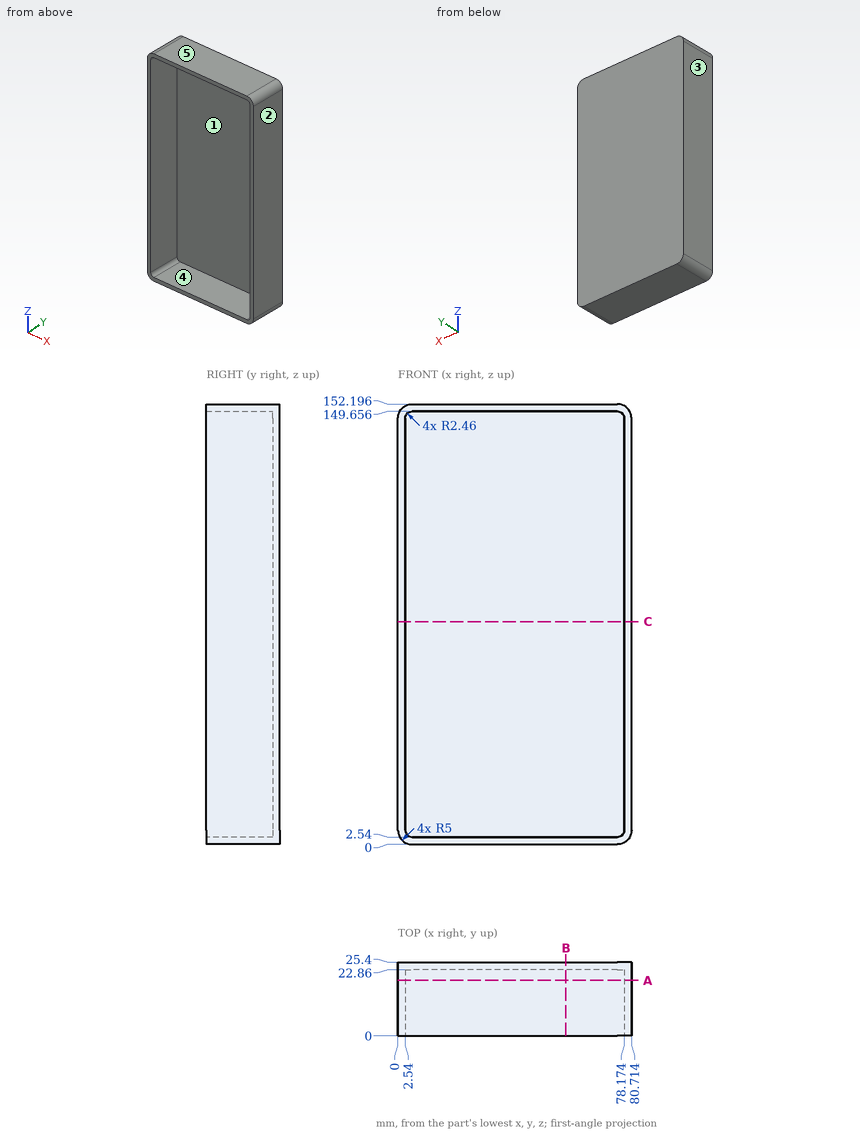
Geometry check sheet. Reference: drawing and pictorial views, mm from the part's lowest x, y, z. A direction names the side the tool comes from. Coordinates: 2 decimals unless noted, no trailing zeros. Write each loop counter-clockwise with the first axis right and the second up, starting at its lowest first coordinate (ties: lowest second). Pieces come first, ordered by that corner, then holes. Notation, with made-up numbers: M -32,18 L 2,18 A21 ccw 2,44 Z; hole C 36.25,15.25 d5. An arc over 180 degrees is marked long. Write item = value, one per line. Start each with the question number.
1. Tool access check on the marked faces 1 and 2. Record the directions out of +Z, -Z, +X, -X, +Y, -Y that give a thin tool (end or side, any length) a straight path to the whole face; none if there is none.
2. Mould release check, pull along Z, two halves, no side actions. Record for the marked faces 3, 4 and 5: pulls with the +Z half, pulls with the -Z half, needs draft (parallel to the pull), parting line crosses it, or undercut.
3. Sectioned sample at A-A (y = 19.25). Record the cut outline in (x, z), then the cut area to 3 significant figures.
4. Sectioned sample at C-C (z = 77). Record the cut outline in (x, y), then the cut area to 3 significant figures.
5. Thickness scan on probe 1 along Z at (x, y) = (30.5, 1.75); probe 2 along X at (y, z) = (22, 40); probe 3 along Y at (x, z) = (48.5, 131.5). Record the ranges inside material, lowest first.
6. Go/stop test with flat-tipped pins: pin 1 (4 mm diameter, centred on x = 50.5, z = 47.5, fed in from -Y); pin 2 (12 mm diameter, centred on y = 20, z = 93, fed in from -X). Record where each tip stops, or that it passes through.
7. Sectioned sample at B-B (x = 58). Record the cut outline in (y, z).
The answers:
q1.face_1 = -Y
q1.face_2 = +Z, -Z, +X, +Y, -Y
q2.face_3 = needs draft
q2.face_4 = undercut
q2.face_5 = pulls with the +Z half
q3.outline = M 0,5 A5 ccw 5,0 L 75.71,0 A5 ccw 80.71,5 L 80.71,147.2 A5 ccw 75.71,152.2 L 5,152.2 A5 ccw 0,147.2 Z; hole M 2.54,5 A2.46 ccw 5,2.54 L 75.71,2.54 A2.46 ccw 78.17,5 L 78.17,147.2 A2.46 ccw 75.71,149.66 L 5,149.66 A2.46 ccw 2.54,147.2 Z
q3.area = 1,140 mm²
q4.outline = M 0,0 L 2.54,0 L 2.54,22.86 L 78.17,22.86 L 78.17,0 L 80.71,0 L 80.71,25.4 L 0,25.4 Z
q4.area = 321 mm²
q5.probe_1 = 0 to 2.54, 149.66 to 152.2
q5.probe_2 = 0 to 2.54, 78.17 to 80.71
q5.probe_3 = 22.86 to 25.4
q6.pin_1 = 22.86
q6.pin_2 = 0
q7.outline = M 0,0 L 25.4,0 L 25.4,152.2 L 0,152.2 L 0,149.66 L 22.86,149.66 L 22.86,2.54 L 0,2.54 Z
